Work out the finished part from the listing and answer in its coordinate system (mm). Face numbers are marked on the shaded views. Coordinates: 2 decimals unless noted, no trailing zeros. Write each loop counter-clockwise with the first axis right and the second up, starting at its lowest first coordinate (ties: lowest second). Pieces come first, ordered by that corner, then holes. Notation, with made-up numbers: (80, 37.25) - (135, 37.25) arc R9 cw to (135, 45.25) - close; hole circle Ø1 at (-32.5, 5). An arc over 180 degrees is marked (long way). Use a Markdown table: item, result. Add a question column.
(1) Find the intervals of material crossed by line 1 (X direction, y = 576.5, z = -1.4); line 2 (Y direction, x = -548.6, z = -1.5); line 3 (X direction, y = 475, z = -14.5), in increasing order. Write a range as from..to.
(2) Given pin 1 Ø1 at (y, z) = (595, -1) entering from -X; pin 2 Ø1.5 at (x, y) = (-125.5, 324.5) entering from -Z; pin 3 Ø0.6 at (x, z) = (-565, -10.5) entering from +Y, each flat-ended and moving along its own axis, determine where each tip first touches the part or whether it passes through.
(3) The part is cut by section C-C, the plane y = 264. Give the vertices of the cut face in (x, z), then the cut area to 3 significant figures.
(4) The part is cut by section A-A, the plane z = -16. Give the vertices of the cut face in (x, y), then the cut area to 3 significant figures.
(5) The part is cut by section B-B, the plane x = -122. Give the vertices of the cut face in (y, z), then the cut area to 3 significant figures.
(6) For a pull along Y with two mould halves and no side action, classify the marked faces 1 and 2 as released by +Y, released by -Y, zero draft, split by the parting line, or undercut.
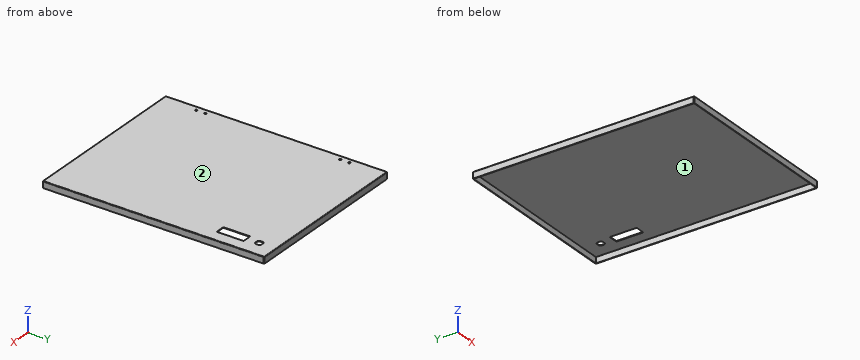
from build123d import *

# Parameters (mm, degrees)
SKIZZE1_W                          = 564
SKIZZE1_H                          = 715.9
BASIS_BLECH_DEPTH                  = 2
KANTE_LASCHE1_DEPTH                = 715.9
KANTE_LASCHE2_DEPTH                = 564
KANTE_LASCHE3_DEPTH                = 715.9
KANTE_LASCHE4_DEPTH                = 564
SCHNITT_LINEAR_AUSTRAGEN1_REACH    = 916.568
F_7_0_7_DURCHMESSER_BOHRUNG1_D     = 7
F_7_0_7_DURCHMESSER_BOHRUNG1_DEPTH = 20
F_7_0_7_DURCHMESSER_BOHRUNG1_TIP   = 2.103012167


# Sheet-metal steps are written as plain solids
with BuildPart() as part:
    # Skizze1 → Basis-Blech (new body)
    with BuildSketch(Plane.XY):
        with Locations((-282, 357.95)):
            Rectangle(SKIZZE1_W, SKIZZE1_H)
    extrude(amount=-BASIS_BLECH_DEPTH)

    # Kante-Lasche1 section (across the edge) → Kante-Lasche1 (add)
    with BuildSketch(Plane(origin=(0.1, 715.9, -2), x_dir=(-1, 0, 0), z_dir=(0, -1, 0))):
        with BuildLine():
            Line((-2, 0.1), (-2, 19))
            Line((-2, 19), (0, 19))
            Line((0, 19), (0, 0.1))
            ThreePointArc((0, 0.1), (0.029289322, 0.029289322), (0.1, 0))
            Line((0.1, 0), (0.1, -2))
            ThreePointArc((0.1, -2), (-1.38492424, -1.38492424), (-2, 0.1))
        make_face()
    extrude(amount=KANTE_LASCHE1_DEPTH)

    # Kante-Lasche2 section (across the edge) → Kante-Lasche2 (add)
    with BuildSketch(Plane(origin=(-564, 716, -2), x_dir=(0, -1, 0), z_dir=(1, 0, 0))):
        with BuildLine():
            Line((-2, 0.1), (-2, 19))
            Line((-2, 19), (0, 19))
            Line((0, 19), (0, 0.1))
            ThreePointArc((0, 0.1), (0.029289322, 0.029289322), (0.1, 0))
            Line((0.1, 0), (0.1, -2))
            ThreePointArc((0.1, -2), (-1.38492424, -1.38492424), (-2, 0.1))
        make_face()
    extrude(amount=KANTE_LASCHE2_DEPTH)

    # Kante-Lasche3 section (across the edge) → Kante-Lasche3 (add)
    with BuildSketch(Plane(origin=(-564.1, 0, -2), x_dir=(1, 0, 0), z_dir=(0, 1, 0))):
        with BuildLine():
            Line((-2, 0.1), (-2, 19))
            Line((-2, 19), (0, 19))
            Line((0, 19), (0, 0.1))
            ThreePointArc((0, 0.1), (0.029289322, 0.029289322), (0.1, 0))
            Line((0.1, 0), (0.1, -2))
            ThreePointArc((0.1, -2), (-1.38492424, -1.38492424), (-2, 0.1))
        make_face()
    extrude(amount=KANTE_LASCHE3_DEPTH)

    # Kante-Lasche4 section (across the edge) → Kante-Lasche4 (add)
    with BuildSketch(Plane(origin=(0, -0.1, -2), x_dir=(0, 1, 0), z_dir=(-1, 0, 0))):
        with BuildLine():
            Line((-2, 0.1), (-2, 19))
            Line((-2, 19), (0, 19))
            Line((0, 19), (0, 0.1))
            ThreePointArc((0, 0.1), (0.029289322, 0.029289322), (0.1, 0))
            Line((0.1, 0), (0.1, -2))
            ThreePointArc((0.1, -2), (-1.38492424, -1.38492424), (-2, 0.1))
        make_face()
    extrude(amount=KANTE_LASCHE4_DEPTH)

    # Skizze17 → Schnitt-Linear austragen1 (cut, up to next)
    with BuildSketch(Plane.XY, mode=Mode.PRIVATE) as schnitt_linear_austragen1_sk1:
        with BuildLine():
            Line((-62.95, 657.944310136), (-62.95, 668.055689864))
            ThreePointArc((-62.95, 668.055689864), (-60.854951288, 670.954951288), (-57.955689864, 673.05))
            Line((-57.955689864, 673.05), (-47.844310136, 673.05))
            ThreePointArc((-47.844310136, 673.05), (-44.945048712, 670.954951288), (-42.85, 668.055689864))
            Line((-42.85, 668.055689864), (-42.85, 657.944310136))
            ThreePointArc((-42.85, 657.944310136), (-44.945048712, 655.045048712), (-47.844310136, 652.95))
            Line((-47.844310136, 652.95), (-57.955689864, 652.95))
            ThreePointArc((-57.955689864, 652.95), (-60.854951288, 655.045048712), (-62.95, 657.944310136))
        make_face()
    schnitt_linear_austragen1_tool1 = extrude(schnitt_linear_austragen1_sk1.sketch, amount=-SCHNITT_LINEAR_AUSTRAGEN1_REACH, mode=Mode.PRIVATE) & part.part
    # Skizze17 → Schnitt-Linear austragen1 (cut, up to next)
    with BuildSketch(Plane.XY, mode=Mode.PRIVATE) as schnitt_linear_austragen1_sk2:
        with BuildLine():
            Line((-66.75, 623), (-39.05, 623))
            ThreePointArc((-39.05, 623), (-37.989339828, 622.560660172), (-37.55, 621.5))
            Line((-37.55, 621.5), (-37.55, 536.9))
            ThreePointArc((-37.55, 536.9), (-37.989339828, 535.839339828), (-39.05, 535.4))
            Line((-39.05, 535.4), (-66.75, 535.4))
            ThreePointArc((-66.75, 535.4), (-67.810660172, 535.839339828), (-68.25, 536.9))
            Line((-68.25, 536.9), (-68.25, 621.5))
            ThreePointArc((-68.25, 621.5), (-67.810660172, 622.560660172), (-66.75, 623))
        make_face()
    schnitt_linear_austragen1_tool2 = extrude(schnitt_linear_austragen1_sk2.sketch, amount=-SCHNITT_LINEAR_AUSTRAGEN1_REACH, mode=Mode.PRIVATE) & part.part
    add(schnitt_linear_austragen1_tool1.solids().sort_by_distance((-52.9, 663, 0))[0], mode=Mode.SUBTRACT)
    add(schnitt_linear_austragen1_tool2.solids().sort_by_distance((-52.9, 579.2, 0))[0], mode=Mode.SUBTRACT)

    # Ø7.0 (7) Durchmesser Bohrung1
    with Locations(Plane.XY):
        with Locations((-548.6, 109.4), (-548.6, 139.4), (-548.6, 576.5), (-548.6, 606.5)):
            Hole(F_7_0_7_DURCHMESSER_BOHRUNG1_D / 2, depth=F_7_0_7_DURCHMESSER_BOHRUNG1_DEPTH)
            with Locations((0, 0, -(F_7_0_7_DURCHMESSER_BOHRUNG1_DEPTH + F_7_0_7_DURCHMESSER_BOHRUNG1_TIP / 2))):  # 118° drill point
                Cone(0, F_7_0_7_DURCHMESSER_BOHRUNG1_D / 2, F_7_0_7_DURCHMESSER_BOHRUNG1_TIP, mode=Mode.SUBTRACT)


solid = part.part
Model answer:
| question | item | result |
|---|---|---|
| 1 | line 1 | -565.98..-552.1, -545.1..-68.25, -37.55..1.98 |
| 1 | line 2 | -2.01..105.9, 112.9..135.9, 142.9..573, 580..603, 610..717.91 |
| 1 | line 3 | -566.1..-564.1, 0.1..2.1 |
| 2 | pin 1 | x = -566.01 |
| 2 | pin 2 | z = -2 |
| 2 | pin 3 | y = 715.9 |
| 3 | outline | (-566.1, -21) - (-564.1, -21) - (-564.1, -2.1) arc R0.1 cw to (-564, -2) - (0, -2) arc R0.1 cw to (0.1, -2.1) - (0.1, -21) - (2.1, -21) - (2.1, -2.1) arc R2.1 ccw to (0, 0) - (-564, 0) arc R2.1 ccw to (-566.1, -2.1) - close |
| 3 | area | 1,210 mm^2 |
| 4 | outline | (-566.1, 0) - (-564.1, 0) - (-564.1, 715.9) - (-566.1, 715.9) - close; (-564, -2.1) - (0, -2.1) - (0, -0.1) - (-564, -0.1) - close; (-564, 716) - (0, 716) - (0, 718) - (-564, 718) - close; (0.1, 0) - (2.1, 0) - (2.1, 715.9) - (0.1, 715.9) - close |
| 4 | area | 5,120 mm^2 |
| 5 | outline | (-2.1, -21) - (-0.1, -21) - (-0.1, -2.1) arc R0.1 cw to (0, -2) - (715.9, -2) arc R0.1 cw to (716, -2.1) - (716, -21) - (718, -21) - (718, -2.1) arc R2.1 ccw to (715.9, 0) - (0, 0) arc R2.1 ccw to (-2.1, -2.1) - close |
| 5 | area | 1,510 mm^2 |
| 6 | face 1 | undercut |
| 6 | face 2 | zero draft |
